Input: part model. Units: mm. Frame: model coordinates. Face numbers are marked on the shaded views. A direction names the side the tool comes from. Round coordinates to 2 decimals unless told otherwise and drop trailing zeros. Loops run counter-clockwise (first coordinate to the right, second up) from the corner with the lowest first, then second, coordinate; pieces in that order, holes last.
(1) Cut plane A-A, the plane y = 0. Output: boundary loops of the cut face in (x, z) (3 decimals).
(2) Access query for the marked faces 1 and 2. Directions: +Z, -Z, +X, -X, +Y, -Y. A direction counts if a zero-diameter tool reaches every point of the face in a straight line with its end or side. Return the directions, or none.
(3) Line query: line 1 (Z direction, x = 0.5, y = 0) (3 decimals); line 2 (Z direction, x = 3, y = 0) (3 decimals); line 3 (Y direction, x = -11, z = -4). Output: solid intervals per line, ascending.
(4) First-contact query: pin 1 Ø8.5 at (y, z) = (0, 0) entering from -X (3 decimals); pin 2 Ø12 at (x, y) = (-3, -29.5) entering from -Z; pin 3 Ø1 at (y, z) = (-32, 23) entering from +X. Flat tips, straight axial feed; report the tip coordinate or a pass-through.
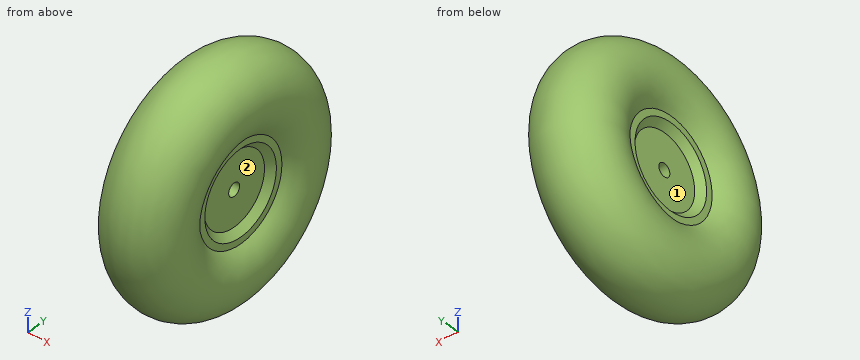
from build123d import *


with BuildPart() as part:
    # Sketch1 → Revolve1 (revolve)
    with BuildSketch(Plane.XY):
        with BuildLine():
            ThreePointArc((-12.7, 23.900968343), (0, 57.15), (12.7, 23.900968343))
            Line((12.7, 23.900968343), (12.7, 20.725968343))
            Line((12.7, 20.725968343), (9.525, 17.550968343))
            Line((9.525, 17.550968343), (9.525, 3.175))
            Line((9.525, 3.175), (-9.525, 3.175))
            Line((-9.525, 3.175), (-9.525, 17.550968343))
            Line((-9.525, 17.550968343), (-12.7, 20.725968343))
            Line((-12.7, 20.725968343), (-12.7, 23.900968343))
        make_face()
    revolve(axis=Axis((-53.506986498, 0, 0), (1, 0, 0)))


solid = part.part
Reported:
1. outline: (-12.7, -23.901) arc R19.05 ccw (long way) to (12.7, -23.901) - (12.7, -20.726) - (9.525, -17.551) - (9.525, -3.175) - (-9.525, -3.175) - (-9.525, -17.551) - (-12.7, -20.726) - close; (-12.7, 20.726) - (-9.525, 17.551) - (-9.525, 3.175) - (9.525, 3.175) - (9.525, 17.551) - (12.7, 20.726) - (12.7, 23.901) arc R19.05 ccw (long way) to (-12.7, 23.901) - close
2. face 1: -X
2. face 2: +X
3. line 1: z = -57.143 to -3.175, 3.175 to 57.143
3. line 2: z = -56.912 to -3.175, 3.175 to 56.912
3. line 3: y = -53.5 to -18.6, 18.6 to 53.5
4. pin 1: stops at x = -9.525
4. pin 2: stops at z = -51.95
4. pin 3: stops at x = 19.03
